from build123d import *

# Parameters (mm, degrees)
SKETCH_1_W                  = 26
SKETCH_1_H                  = 54
SKETCH_1_W_2                = 20
SKETCH_1_H_2                = 40
EXTRUDE_1_DEPTH             = 5
EXTRUDE_2_DEPTH             = 28
SKETCH_3_OUTSIDE_W          = 41.47
SKETCH_3_OUTSIDE_H          = 70.936
CUT_EXTRUDE_1_DEPTH         = 29
FILLET_1_R                  = 5
EXTRUDE_3_DEPTH             = 6
M3X0_51_D                   = 2.5
M3X0_51_CSINK_D             = 3.05
M3X0_51_CSINK_ANGLE         = 90
PATTERN_LINEAR_1_COUNT      = 2
PATTERN_LINEAR_1_PITCH      = 10
PATTERN_LINEAR_1_COUNT_DIR2 = 2
PATTERN_LINEAR_1_PITCH_DIR2 = 48
HOLE_WIZARD_1_D             = 2.5
PATTERN_CIRCULAR_1_COUNT    = 8


with BuildPart() as part:
    # Эскиз1 → Бобышка-Вытянуть1 (new body)
    with BuildSketch(Plane.XY):
        with Locations((0, -10)):
            Rectangle(SKETCH_1_W, SKETCH_1_H)
        with Locations((0, -10)):
            Rectangle(SKETCH_1_W_2, SKETCH_1_H_2, mode=Mode.SUBTRACT)
    extrude(amount=EXTRUDE_1_DEPTH)

    # Эскиз2 → Бобышка-Вытянуть2 (add)
    with BuildSketch(Plane.XY):
        with BuildLine():
            Line((10, -18.466185313), (10, 18.466185313))
            ThreePointArc((10, 18.466185313), (11.542267321, 17.543547677), (13, 16.492422502))
            Line((13, 16.492422502), (13, -16.492422502))
            ThreePointArc((13, -16.492422502), (11.542267321, -17.543547677), (10, -18.466185313))
        make_face()
        with BuildLine():
            Line((-10, -18.466185313), (-10, 18.466185313))
            ThreePointArc((-10, 18.466185313), (-11.542267321, 17.543547677), (-13, 16.492422502))
            Line((-13, 16.492422502), (-13, -16.492422502))
            ThreePointArc((-13, -16.492422502), (-11.542267321, -17.543547677), (-10, -18.466185313))
        make_face()
    extrude(amount=EXTRUDE_2_DEPTH)

    # Эскиз3 outside → Вырез-Вытянуть1 (cut, through all)
    with BuildSketch(Plane.XY.offset(28)):
        with Locations((0, -9.267)):
            Rectangle(SKETCH_3_OUTSIDE_W, SKETCH_3_OUTSIDE_H)
        with BuildLine():
            Line((-13, -16.492422502), (-13, -37))
            Line((-13, -37), (13, -37))
            Line((13, -37), (13, -16.492422502))
            ThreePointArc((13, -16.492422502), (0, 21), (-13, -16.492422502))
        make_face(mode=Mode.SUBTRACT)
    extrude(amount=-CUT_EXTRUDE_1_DEPTH, mode=Mode.SUBTRACT)

    # Скругление1
    fillet_1_edges = [part.edges().sort_by_distance(p)[0] for p in [
        (13, -37, 2.5),
        (-13, -37, 2.5),
    ]]
    fillet(fillet_1_edges, radius=FILLET_1_R)

    # Эскиз7 → Бобышка-Вытянуть3 (add)
    with BuildSketch(Plane.XY.offset(28)):
        with BuildLine():
            Line((-10, -22.912878475), (-10, 22.912878475))
            ThreePointArc((-10, 22.912878475), (-25, 0), (-10, -22.912878475))
        make_face()
        with BuildLine():
            Line((10, -22.912878475), (10, 22.912878475))
            ThreePointArc((10, 22.912878475), (25, 0), (10, -22.912878475))
        make_face()
    extrude(amount=EXTRUDE_3_DEPTH)

    # Отверстие обработанное метчиком M3x0.51 (through all)
    with Locations(Plane.XY.offset(5)):
        with Locations((-5, 14)):
            m3x0_51 = CounterSinkHole(M3X0_51_D / 2, M3X0_51_CSINK_D / 2, counter_sink_angle=M3X0_51_CSINK_ANGLE)

    # Линейный массив1: M3x0.51 2 × 2
    with Locations(*[(i * PATTERN_LINEAR_1_PITCH, -j * PATTERN_LINEAR_1_PITCH_DIR2, 0) for i in range(PATTERN_LINEAR_1_COUNT) for j in range(PATTERN_LINEAR_1_COUNT_DIR2) if (i, j) != (0, 0)]):
        add(m3x0_51, mode=Mode.SUBTRACT)

    # Отверстие1 (through all)
    with Locations(Plane.XY.offset(34)):
        with Locations((-23, 0)):
            hole_wizard_1 = Hole(HOLE_WIZARD_1_D / 2)

    # Круговой массив1: Отверстие1 ×8 about axis, 4 skipped
    pattern_circular_1_axis = Axis((0, 0, 34), (0, 0, 1))
    add([hole_wizard_1.rotate(pattern_circular_1_axis, i * 360 / PATTERN_CIRCULAR_1_COUNT) for i in range(1, PATTERN_CIRCULAR_1_COUNT) if i not in (1, 2, 3, 6)], mode=Mode.SUBTRACT)


solid = part.part
Verification items for the finished model (mm, model axes). A direction names the side the tool comes from. Coordinates: 2 decimals unless noted, no trailing zeros. Loops run counter-clockwise (first coordinate to the right, second up) from the corner with the lowest first, then second, coordinate; pieces in that order, holes last. Notation, with made-up numbers: (15, 79) -> (47, 79) arc R21 ccw to (47, 88) -> close; hole circle Ø3 at (-33.75, -32). An arc over 180 degrees is marked (long way). Answer as a JSON object with one key per item and string values. Group by question number.
Item 1: Depth check by flat-ended pin: pin 1 (10 mm diameter, centred on x = -3, z = 30.5, fed in from +Y); pin 2 (12 mm diameter, centred on x = -20, y = -7, fed in from -Z); pin 3 (3.5 mm diameter, centred on x = -1, y = 12.5, fed in from +Z); pin 4 (4 mm diameter, centred on x = -5, z = 2, fed in from +Y). Enter the tip coordinate at first touch or a pass-through.
Item 2: Sectioned sample at A-A on y = 7. Record the boundary of the cut face in (x, z), plus the area to 3 significant figures.
Item 3: Tool access check on faces 4 (the cylindrical face through (-12, -35, 3)), 5 (the cylindrical face through (-11.52, 17.56, 14.2)), 6 (the flat face through (0, 10, 2)), 7 (the cylindrical face through (12, -35, 3)), 8 (the flat face through (13, -3, 14)). Record the directions out of +Z, -Z, +X, -X, +Y, -Y that give a thin tool (end or side, any length) a straight path to the whole face; none if there is none.
Item 4: Mould release check, pull along X, two halves, no side actions. Record for faces 1 (the flat face through (0, 14, 5)), 2 (the cylindrical face through (-11.56, -17.53, 16.34)), 3 (the cylindrical face through (11.52, 17.56, 13.8)): +X half, -X half, draft (parallel to the pull), parting line (faces both ways), or undercut.
Item 5: Sectioned sample at C-C on z = 4. Record the boundary of the cut face in (x, y), plus the area to 3 significant figures.
Item 6: Scan lines: probe 1 along Y at (x, z) = (-5, 1.7); probe 2 along X at (y, z) = (-7, 10); probe 3 along Y at (x, z) = (23, 30.3). Record each from-to range of solid material in increasing order.
Item 7: Sectioned sample at D-D on z = 15. Record the boundary of the cut face in (x, y).
Item 8: Sectioned sample at B-B on x = 5. Record the boundary of the cut face in (y, z) (3 decimals), plus the area to 3 significant figures.
Evaluation:
{
 "1": {"pin 1": "passes through", "pin 2": "stops at z = 28", "pin 3": "stops at z = 5", "pin 4": "stops at y = 17"},
 "2": {"outline": "(-24, 28) -> (-13, 28) -> (-13, 0) -> (-10, 0) -> (-10, 34) -> (-24, 34) -> close; (10, 0) -> (13, 0) -> (13, 28) -> (24, 28) -> (24, 34) -> (10, 34) -> close", "area": "336 mm²"},
 "3": {"face 4": "+Z, -Z, -X, -Y", "face 5": "-Z, -X, +Y", "face 6": "+Z, -Z", "face 7": "+Z, -Z, +X, -Y", "face 8": "-Z, +X, +Y, -Y"},
 "4": {"face 1": "undercut", "face 2": "-X half", "face 3": "+X half"},
 "5": {"outline": "(-13, -32) arc R5 ccw to (-8, -37) -> (8, -37) arc R5 ccw to (13, -32) -> (13, 16.49) arc R21 ccw to (10, 18.47) -> (10, 17) -> (-10, 17) -> (-10, 18.47) arc R21 ccw to (-13, 16.49) -> close; hole (-10, -30) -> (10, -30) -> (10, 10) -> (-10, 10) -> close; hole circle Ø2.5 at (-5, -34); hole circle Ø2.5 at (-5, 14); hole circle Ø2.5 at (5, -34); hole circle Ø2.5 at (5, 14)", "area": "577 mm²"},
 "6": {"probe 1": "y = -37 to -35.25, -32.75 to -30, 10 to 12.75, 15.25 to 17", "probe 2": "x = -13 to -10, 10 to 13", "probe 3": "y = -9.8 to -1.25, 1.25 to 9.8"},
 "7": {"outline": "(-13, -16.49) arc R21 ccw to (-10, -18.47) -> (-10, 18.47) arc R21 ccw to (-13, 16.49) -> close; (10, -18.47) arc R21 ccw to (13, -16.49) -> (13, 16.49) arc R21 ccw to (10, 18.47) -> close"},
 "8": {"outline": "(-37, 0) -> (-35.25, 0) -> (-35.25, 4.725) -> (-35.525, 5) -> (-37, 5) -> close; (-32.75, 0) -> (-30, 0) -> (-30, 5) -> (-32.475, 5) -> (-32.75, 4.725) -> close; (10, 0) -> (12.75, 0) -> (12.75, 4.725) -> (12.475, 5) -> (10, 5) -> close; (15.25, 0) -> (17, 0) -> (17, 5) -> (15.525, 5) -> (15.25, 4.725) -> close", "area": "44.8 mm²"}
}
